```python
from build123d import *

# Parameters (mm, degrees)
F3_DEPTH = 1016
F4_W     = 1600.2
F4_H     = 19.05
F5_DEPTH = 736.6


with BuildPart() as f3:
    # F2 (on Front) → F3 (new body)
    with BuildSketch(Plane.XZ):
        Polygon((0, 762), (0, 0), (25.4, 0), (25.4, 736.6), align=None)
        Polygon((1651, 762), (0, 762), (25.4, 736.6), (1625.6, 736.6), align=None)
        Polygon((1651, 0), (1651, 762), (1625.6, 736.6), (1625.6, 0), align=None)
    extrude(amount=F3_DEPTH)

    # F4 (on face) → F5 (join, through all)
    with BuildSketch(Plane(origin=(0, 0, 736.6), x_dir=(1, 0, 0), z_dir=(0, 0, -1))):
        with Locations((825.5, 677.3333333333)):
            Rectangle(F4_W, F4_H)
    extrude(amount=F5_DEPTH)


solid = f3.part
```
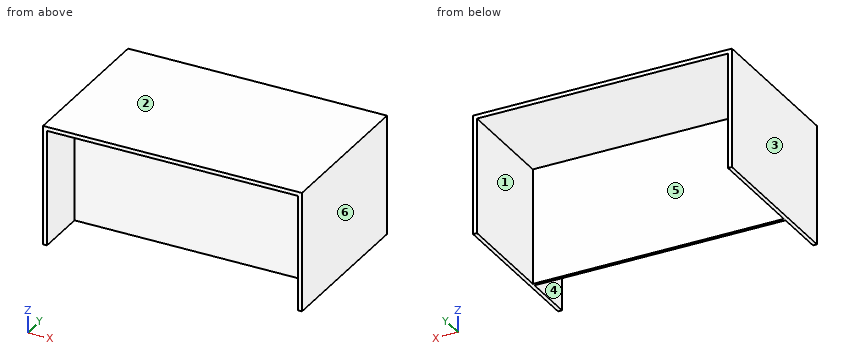
For this review, take the finished solid that the model builds, in its own axes (mm). Face numbers are marked on the shaded views. A direction names the side the tool comes from. Coordinates: 2 decimals unless noted, no trailing zeros. Loops run counter-clockwise (first coordinate to the right, second up) from the corner with the lowest first, then second, coordinate; pieces in that order, holes last.
1. For line 1 (X direction, y = -510, z = 389); line 2 (Y direction, x = 1576, z = 160); line 3 (Z direction, x = 1108.5, y = -750.5), list the stretches that pass through material, from the lowest coordinate up.
2. For the marked faces 4, 5 and 6, list the 3-axis set-ups (+Z, -Z, +X, -X, +Y, -Y) from which the entire face can be reached by the end or side of a thin tool; tool diameter is ignored.
3. Add section A-A, the plane x = 1181. Give the boundary of the cut face in (y, z).
4. Add section B-B, the plane y = -937. Give the boundary of the cut face in (x, z).
5. Mouldability with a two-part tool opening along X and no side actions: class the marked faces 1, 2 and 3 as +X half, -X half, draft (parallel to the pull), parting line (faces both ways), or undercut.
6. Insertion check: P1, Ø5, axis at x = 1083.5, y = -868.5, coming from the -Z side; P2, Ø2, axis at x = 897, z = 334, coming from the -Y side; P3, Ø2, axis at x = 329, z = 235.5, coming from the +Y side. Each pin has a flat end and moves straight along its axis. Give the tip position at first contact, or say it passes through.
7. Add section C-C, the plane z = 464. Give the boundary of the cut face in (x, y), then the cut area to 3 significant figures.
Result:
1. line 1: x = 0 to 25.4, 1625.6 to 1651
1. line 2: y = -686.86 to -667.81
1. line 3: z = 736.6 to 762
2. face 4: -Z, -Y
2. face 5: -Z, +Y
2. face 6: +Z, -Z, +X, +Y, -Y
3. outline: (-1016, 736.6) - (-686.86, 736.6) - (-686.86, 0) - (-667.81, 0) - (-667.81, 736.6) - (0, 736.6) - (0, 762) - (-1016, 762) - close
4. outline: (0, 0) - (25.4, 0) - (25.4, 736.6) - (1625.6, 736.6) - (1625.6, 0) - (1651, 0) - (1651, 762) - (0, 762) - close
5. face 1: undercut
5. face 2: draft
5. face 3: -X half
6. P1: stops at z = 736.6
6. P2: stops at y = -686.86
6. P3: stops at y = -667.81
7. outline: (0, -1016) - (25.4, -1016) - (25.4, -686.86) - (1625.6, -686.86) - (1625.6, -1016) - (1651, -1016) - (1651, 0) - (1625.6, 0) - (1625.6, -667.81) - (25.4, -667.81) - (25.4, 0) - (0, 0) - close
7. area: 82,100 mm2
